Autodesk Inventor part; units mm, degrees
ref_plane "YZ Plane" through (0, 0, 0) normal (1, 0, 0) x (0, 1, 0)
ref_plane "XZ Plane" through (0, 0, 0) normal (0, 1, 0) x (-1, 0, 0)
ref_plane "XY Plane" through (0, 0, 0) normal (0, 0, 1) x (1, 0, 0)
sketch "スケッチ1" plane through (0, 0, 0) normal (0, 0, 1) x (1, 0, 0)
  line L0 (10, -10) -> (-10, -10)
  line L1 (-10, -10) -> (-10, 10)
  line L2 (-10, 10) -> (10, 10)
  line L3 (10, 10) -> (10, -10)
  line L4 (10, -10) -> (-10, 10) construction
  line L5 (-10, -10) -> (10, 10) construction
  line L6 (9, 9) -> (-9, 9)
  line L7 (-9, 9) -> (-9, -9)
  line L8 (-9, -9) -> (9, -9)
  line L9 (9, -9) -> (9, 9)
  point P0 (0, 0)
  dimension "d0" = 20
  dimension "d1" = 20
  dimension "d2" = 1
extrude "押し出し1" add sketch "スケッチ1" along normal blind 300
sketch "スケッチ2" plane through (10, -10, 0) normal (1, 0, 0) x (0, 0, -1)
  line L0 (0, 10) -> (-300, 10)
  line L1 (-300, 0) -> (-300, 20)
  line L2 (0, 0) -> (0, 20)
  point P0 (-290, 10)
  point P1 (-10, 10)
  point P2 (-150, 10)
  point P3 (-170, 10)
  point P4 (-130, 10)
  dimension "d5" = 10
  dimension "d6" = 10
  dimension "d17" = 20
  dimension "d18" = 20
hole "穴1" at (10, 0, 290) at (10, 0, 10) at (10, 0, 170) at (10, 0, 130) direction (-1, 0, 0) diameter 3.2 end through all
sketch "スケッチ3" plane through (10, -10, 0) normal (1, 0, 0) x (0, 0, -1)
  line L0 (0, 10) -> (-300, 10)
  line L1 (-300, 1) -> (-300, 19)
  circle A0 centre (-150, 10) radius 6
  dimension "d14" = 12
extrude "押し出し2" cut sketch "スケッチ3" against normal blind 300
properties part number "xx_shita"
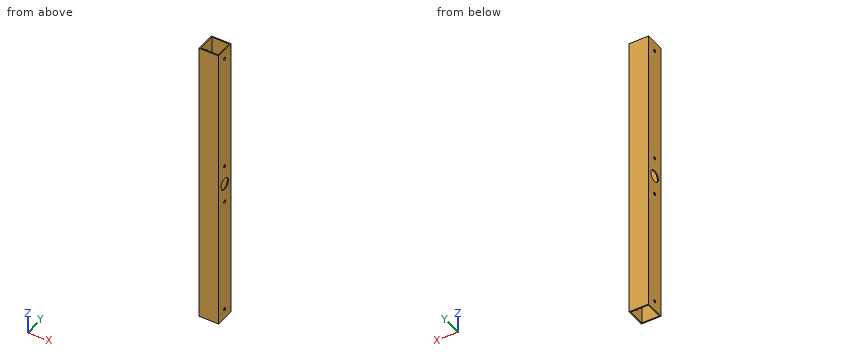
Geometry: final body of the model. Coordinates: model frame, mm. Coordinates: 2 decimals unless noted, no trailing zeros. Order: outer loops, then holes, each group sorted by start corner. A loop starts at its lowest first (then second) coordinate and runs counter-clockwise, first axis right, second up. Notation, with made-up numbers: (77.25, -23.5) -> (124.25, -23.5) arc R22 ccw to (124.25, -11.5) -> close; hole circle Ø4 at (28.25, 23). An arc over 180 degrees is marked (long way). Answer in a Markdown table with one row per item.
Item 1: Section B-B on z = 278.5. Output: boundary loops of the cut face in (x, y).
Return value:
| item | result |
|---|---|
| outline | (-10, -10) -> (10, -10) -> (10, 10) -> (-10, 10) -> close; hole (-9, -9) -> (9, -9) -> (9, 9) -> (-9, 9) -> close |
Item 2: Ray query, L1, parallel to Z at x = 9.45, y = 0; L2, parallel to X at y = 7.25, z = 146. Return the intervals inside material, ascending.
Return value:
| item | result |
|---|---|
| L1 | z = 0 to 8.4, 11.6 to 128.4, 131.6 to 144, 156 to 168.4, 171.6 to 288.4, 291.6 to 300 |
| L2 | x = -10 to -9, 9 to 10 |
Item 3: Section A-A on x = -4.5. Output: boundary loops of the cut face in (y, z), plus the area to 3 significant figures.
Return value:
| item | result |
|---|---|
| outline | (-10, 0) -> (-9, 0) -> (-9, 300) -> (-10, 300) -> close; (9, 0) -> (10, 0) -> (10, 300) -> (9, 300) -> close |
| area | 600 mm² |
